Source: CAD feature listing. Evaluate the final solid. Frame: model axes, mm. A direction names the side the tool comes from. Give positions to 0.01 mm unless a question says otherwise; leave off trailing zeros. Order: outer loops, then holes, each group sorted by start corner. A loop starts at its lowest first (then second) coordinate and runs counter-clockwise, first axis right, second up. Notation, with made-up numbers: M 38.25,1.25 L 56.25,1.25 A21 cw 56.25,5.25 Z; hole C 19,46.5 d10. An arc over 180 degrees is marked long. Use CSV: the item, a comma, the result in double quotes. Start each with the question number.
1. Section query A-A, the plane x = 42. Return the cut outline in (y, z).
2. Reachability of faces 5 (the flat face through (57, 0, -5)), 6 (the cylindrical face through (83.933, 1.014, -5.057)) from +Z, -Z, +X, -X, +Y, -Y: full face, straight path, thin tool, end or side. Return the list, or none.
3. Mould query, pull axis X, two halves, no side actions, for faces 1 (the cylindrical face through (24.6, 1, -5.1)), 2 (the flat face through (57, 2, -5)), 3 (the flat face through (73, 1, -2.4)), 4 (the flat face through (115, 1, -2)). Classes: released by +X, released by -X, zero draft, split by the parting line, or undercut.
4. Line query: line 1 along X through (y, z) = (1.5, -5); line 2 along Z through (x, y) = (69.5, 0.6); line 3 along X through (y, z) = (1.2, -4.25). Output: solid intervals per line, ascending. Write a range as [from, to].
5. Section query B-B, the plane y = 1.6. Return the cut outline in (x, z).
6. Section query C-C, the plane z = -5. Return the cut outline in (x, y).
from build123d import *

# Parameters (mm, degrees)
SKETCH_1_W          = 116
SKETCH_1_H          = 10
EXTRUDE_1_DEPTH     = 2
CUT_EXTRUDE_1_DEPTH = 10
CHAMFER_1_SIZE      = 3


with BuildPart() as part:
    # 스케치1 → 보스-돌출1 (new body)
    with BuildSketch(Plane(origin=(0, 0, 0), x_dir=(1, 0, 0), z_dir=(0, 1, 0))):
        with Locations((58, 5)):
            Rectangle(SKETCH_1_W, SKETCH_1_H)
    extrude(amount=EXTRUDE_1_DEPTH)

    # 스케치2 → 컷-돌출1 (cut)
    with BuildSketch(Plane(origin=(0, 2, 0), x_dir=(1, 0, 0), z_dir=(0, 1, 0))):
        with BuildLine():
            Line((5, 7.6), (22, 7.6))
            ThreePointArc((22, 7.6), (24.6, 5), (22, 2.4))
            Line((22, 2.4), (5, 2.4))
            ThreePointArc((5, 2.4), (2.4, 5), (5, 7.6))
        make_face()
        with BuildLine():
            Line((34.666666667, 7.6), (51.666666667, 7.6))
            ThreePointArc((51.666666667, 7.6), (54.266666667, 5), (51.666666667, 2.4))
            Line((51.666666667, 2.4), (34.666666667, 2.4))
            ThreePointArc((34.666666667, 2.4), (32.066666667, 5), (34.666666667, 7.6))
        make_face()
        with BuildLine():
            Line((64.333333333, 7.6), (81.333333333, 7.6))
            ThreePointArc((81.333333333, 7.6), (83.933333333, 5), (81.333333333, 2.4))
            Line((81.333333333, 2.4), (64.333333333, 2.4))
            ThreePointArc((64.333333333, 2.4), (61.733333333, 5), (64.333333333, 7.6))
        make_face()
        with BuildLine():
            Line((94, 7.6), (111, 7.6))
            ThreePointArc((111, 7.6), (113.6, 5), (111, 2.4))
            Line((111, 2.4), (94, 2.4))
            ThreePointArc((94, 2.4), (91.4, 5), (94, 7.6))
        make_face()
    extrude(amount=-CUT_EXTRUDE_1_DEPTH, mode=Mode.SUBTRACT)

    # 모따기1
    chamfer_1_edges = [part.edges().sort_by_distance(p)[0] for p in [
        (116, 1, 0),
        (0, 1, 0),
    ]]
    chamfer(chamfer_1_edges, length=CHAMFER_1_SIZE)


solid = part.part
Result set:
1,outline,"M 0,-10 L 2,-10 L 2,-7.6 L 0,-7.6 Z; M 0,-2.4 L 2,-2.4 L 2,0 L 0,0 Z"
2,face 5,"+Z, -Z, +X, -X, -Y"
2,face 6,"+Y, -Y"
3,face 1,"undercut"
3,face 2,"zero draft"
3,face 3,"undercut"
3,face 4,"released by +X"
4,line 1,"[0, 2.4], [24.6, 32.07], [54.27, 61.73], [83.93, 91.4], [113.6, 116]"
4,line 2,"[-10, -7.6], [-2.4, 0]"
4,line 3,"[0, 2.51], [24.49, 32.18], [54.16, 61.84], [83.82, 91.51], [113.49, 116]"
5,outline,"M 0,-10 L 116,-10 L 116,-3 L 113,0 L 3,0 L 0,-3 Z; hole M 5,-7.6 L 22,-7.6 A2.6 ccw 22,-2.4 L 5,-2.4 A2.6 ccw Z; hole M 34.67,-7.6 L 51.67,-7.6 A2.6 ccw 51.67,-2.4 L 34.67,-2.4 A2.6 ccw Z; hole M 64.33,-7.6 L 81.33,-7.6 A2.6 ccw 81.33,-2.4 L 64.33,-2.4 A2.6 ccw Z; hole M 94,-7.6 L 111,-7.6 A2.6 ccw 111,-2.4 L 94,-2.4 A2.6 ccw Z"
6,outline,"M 0,0 L 2.4,0 L 2.4,2 L 0,2 Z; M 24.6,0 L 32.07,0 L 32.07,2 L 24.6,2 Z; M 54.27,0 L 61.73,0 L 61.73,2 L 54.27,2 Z; M 83.93,0 L 91.4,0 L 91.4,2 L 83.93,2 Z; M 113.6,0 L 116,0 L 116,2 L 113.6,2 Z"
